Work out the finished part from the listing and answer in its coordinate system (mm). A direction names the side the tool comes from. Round coordinates to 2 decimals unless told otherwise and drop trailing zeros. Order: outer loops, then holes, each group sorted by start corner. A loop starts at its lowest first (then second) coordinate and runs counter-clockwise, first axis right, second up. Notation, with made-up numbers: (41, 3) - (75, 3) arc R8 ccw to (75, 13) - close; hole circle Ø9 at (58.25, 77.5). An arc over 180 degrees is marked (long way). Use CSV: the item, a comma, the result in double quotes.
from build123d import *

# Parameters (mm, degrees)
F1_DEPTH = 3
F2_DEPTH = 1.4


with BuildPart() as f1:
    # F0 (on Top) → F1 (new body)
    with BuildSketch(Plane.XY):
        with BuildLine():
            Line((-76.5, 36), (-71.383327, 36))
            Line((-71.383327, 36), (-71.383327, 43))
            Line((-71.383327, 43), (-92.759609, 43))
            Line((-92.759609, 43), (-92.759609, -43))
            Line((-92.759609, -43), (-71.383327, -43))
            Line((-71.383327, -43), (-71.383327, -36))
            Line((-71.383327, -36), (-76.5, -36))
            Line((-76.5, -36), (-84.5, -36))
            ThreePointArc((-84.5, -36), (-87.914214, -37.414214), (-86.5, -34))
            Line((-86.5, -34), (-86.5, -26))
            Line((-86.5, -26), (-86.5, 26))
            Line((-86.5, 26), (-86.5, 34))
            ThreePointArc((-86.5, 34), (-87.914214, 37.414214), (-84.5, 36))
            Line((-84.5, 36), (-76.5, 36))
        make_face()
        with BuildLine():
            ThreePointArc((-86.5, 26), (-83.571068, 33.071068), (-76.5, 36))
            Line((-76.5, 36), (-84.5, 36))
            ThreePointArc((-84.5, 36), (-85.085786, 34.585786), (-86.5, 34))
            Line((-86.5, 34), (-86.5, 26))
        make_face()
        with BuildLine():
            Line((-84.5, -36), (-76.5, -36))
            ThreePointArc((-76.5, -36), (-83.571068, -33.071068), (-86.5, -26))
            Line((-86.5, -26), (-86.5, -34))
            ThreePointArc((-86.5, -34), (-85.085786, -34.585786), (-84.5, -36))
        make_face()
    extrude(amount=F1_DEPTH)

    # F0 (on Top) → F2 (join)
    with BuildSketch(Plane.XY):
        with BuildLine():
            Line((-71.383327, -36), (-71.383327, 36))
            Line((-71.383327, 36), (-76.5, 36))
            ThreePointArc((-76.5, 36), (-83.571068, 33.071068), (-86.5, 26))
            Line((-86.5, 26), (-86.5, -26))
            ThreePointArc((-86.5, -26), (-83.571068, -33.071068), (-76.5, -36))
            Line((-76.5, -36), (-71.383327, -36))
        make_face()
    extrude(amount=F2_DEPTH)


solid = f1.part
(1) For faces 1 (the flat face through (-74, 36, 2)), 2 (the flat face through (-71.383, -1, 1)), determine the directions among +Z, -Z, +X, -X, +Y, -Y from which every point of the face is accessible in a straight line to the end or side of a thin tool.
Findings below:
face 1,"+Z, +X"
face 2,"+Z, -Z, +X, +Y, -Y"
(2) Each of these flat-tipped pins is pushed along its axis until it touches: pin 1 (0.8 mm diameter, centred on y = 4, z = 2.5, fed in from +X); pin 2 (12 mm diameter, centred on x = -78.5, y = -5, fed in from +Z); pin 3 (3 mm diameter, centred on x = -86.5, y = 36, fed in from -Z). Where does it stop, or does it pass through?
Findings below:
pin 1,"stops at x = -86.5"
pin 2,"stops at z = 1.4"
pin 3,"passes through"
(3) The mould has two halves that part along Y. Classify faces 3 (the cylindrical face through (-83.49, -33.15, 2.19)), 4 (the flat face through (-82, 1, 0)), 5 (the flat face through (-82, -43, 1)), 6 (the flat face through (-82, 43, 1)): released by +Y, released by -Y, zero draft, split by the parting line, or undercut.
Findings below:
face 3,"undercut"
face 4,"zero draft"
face 5,"released by -Y"
face 6,"released by +Y"
(4) Find section A-A (z = 2.45). Determine the outline of the cut face in (x, y), and give its area (3 significant figures).
Findings below:
outline,"(-92.76, -43) - (-71.38, -43) - (-71.38, -36) - (-76.5, -36) arc R10 cw to (-86.5, -26) - (-86.5, 26) arc R10 cw to (-76.5, 36) - (-71.38, 36) - (-71.38, 43) - (-92.76, 43) - close; hole (-86.5, -34) arc R2 ccw (long way) to (-84.5, -36) arc R2 ccw to start; hole (-86.5, 34) arc R2 ccw to (-84.5, 36) arc R2 ccw (long way) to start"
area,"768 mm²"
(5) Find the intervals of material crossed by L1, parallel to Y at x = -86.5, z = 0.85; L2, parallel to Y at x = -75.25, z = 2.9; L3, parallel to Y at x = -85.75, z = 0.85, in increasing order. Write a range as from..to.
Findings below:
L1,"y = -43..-38, -34..34, 38..43"
L2,"y = -43..-36, 36..43"
L3,"y = -43..-37.85, -34.15..34.15, 37.85..43"
(6) Find section D-D (x = -79.5). Determine the outline of the cut face in (y, z).
Findings below:
outline,"(-43, 0) - (43, 0) - (43, 3) - (35.54, 3) - (35.54, 1.4) - (-35.54, 1.4) - (-35.54, 3) - (-43, 3) - close"
(7) Find section B-B (x = -75). Determine the outline of the cut face in (y, z).
Findings below:
outline,"(-43, 0) - (43, 0) - (43, 3) - (36, 3) - (36, 1.4) - (-36, 1.4) - (-36, 3) - (-43, 3) - close"
(8) Find section C-C (y = -21). Determine the outline of the cut face in (x, z).
Findings below:
outline,"(-92.76, 0) - (-71.38, 0) - (-71.38, 1.4) - (-86.5, 1.4) - (-86.5, 3) - (-92.76, 3) - close"
